Can you work these out from the drawing? Everything is in mm from the part's minimum corner. Give positions to 0.01 mm unless a question says otherwise; leave off trailing zeros. Loops run counter-clockwise (first coordinate to the right, second up) from the corner with the lowest first, then second, coordinate; pieces in that order, holes last. Notation, with made-up numbers: (-23.5, -19.5) -> (11.5, -19.5) arc R35 ccw to (11.5, 16.5) -> close; hole circle Ø3 at (5.5, 37). An arc over 180 degrees is marked (long way). Return JSON: item names as keys, results as strings. Group by question number.
Q1. Will these pins go through, and if not, where does the flat tip stop? pin 1 (3 mm diameter, centred on x = 9, y = 9, fed in from -Z); pin 2 (1.8 mm diameter, centred on x = 14.63, y = 5.75, fed in from +Z); pin 3 (3 mm diameter, centred on x = 12.5, z = 4, fed in from -Y) (3 decimals); pin 4 (3 mm diameter, centred on x = 6, z = 1.5, fed in from +Y).
Q2. Suppose I cut it at D-D, the plane y = 13.25. Please give me the cut outline in (x, z).
Q3. I need wall thicknesses on line 1 along Y through (x, z) = (9, 6.75); line 2 along X through (y, z) = (5.25, 6) (1 decimal); line 3 along X through (y, z) = (1.75, 4.5). Which ranges of each line are inside material? Lowest first, please. Write a range as [from, to].
Q4. Suppose I cut it at B-B, the plane y = 9. Please give me the cut outline in (x, z).
Q5. Thinking about a two-plate mould opening in Y: for the marked faces 1, 2 and 3, which applies, pulls with the +Y half, pulls with the -Y half, needs draft (parallel to the pull), parting line crosses it, or undercut?
Q6. Suppose I cut it at C-C, the plane z = 7. Please give me the cut outline in (x, y).
Q7. Suppose I cut it at A-A, the plane x = 9. Please give me the cut outline in (y, z), and give its area (3 significant figures).
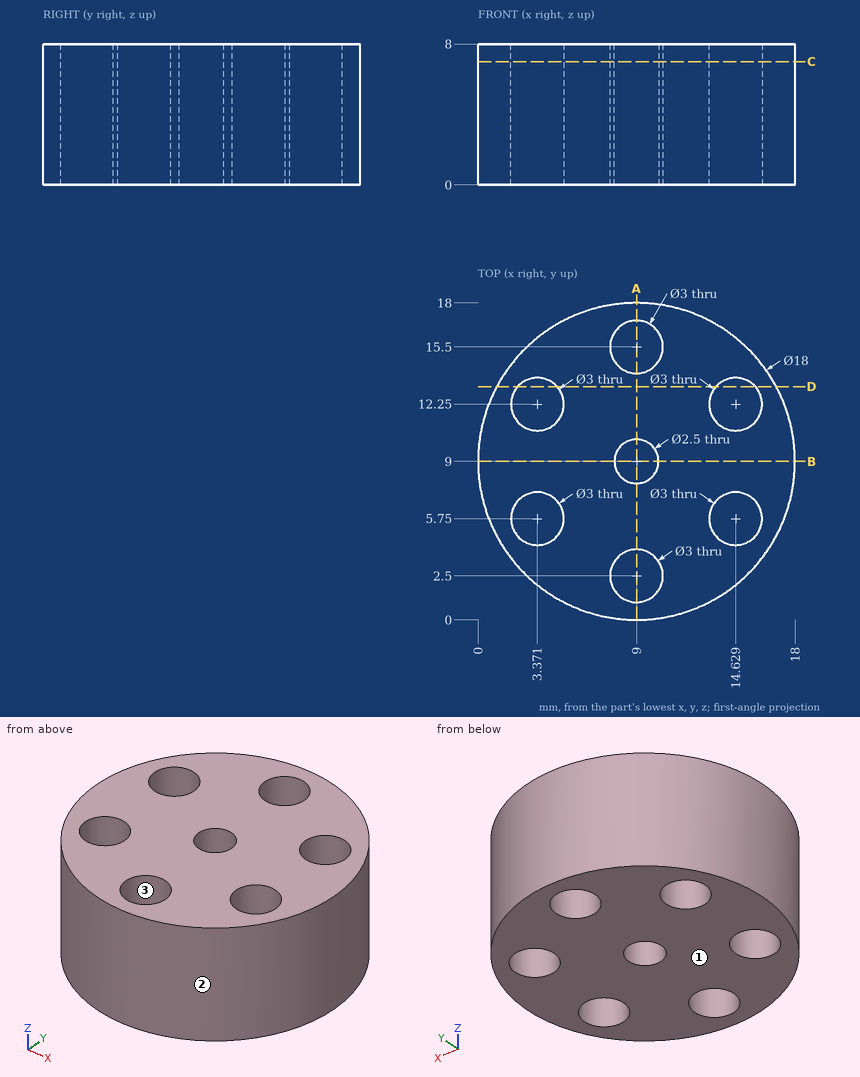
Ans:
{
 "1": {"pin 1": "stops at z = 0", "pin 2": "passes through", "pin 3": "stops at y = 0.225", "pin 4": "stops at y = 17.87"},
 "2": {"outline": "(1.07, 0) -> (2.25, 0) -> (2.25, 8) -> (1.07, 8) -> close; (4.49, 0) -> (13.51, 0) -> (13.51, 8) -> (4.49, 8) -> close; (15.75, 0) -> (16.93, 0) -> (16.93, 8) -> (15.75, 8) -> close"},
 "3": {"line 1": "y = [0, 1], [4, 7.75], [10.25, 14], [17, 18]", "line 2": "x = [0.8, 2], [4.8, 13.2], [16, 17.2]", "line 3": "x = [3.67, 7.7], [10.3, 14.33]"},
 "4": {"outline": "(0, 0) -> (7.75, 0) -> (7.75, 8) -> (0, 8) -> close; (10.25, 0) -> (18, 0) -> (18, 8) -> (10.25, 8) -> close"},
 "5": {"face 1": "needs draft", "face 2": "parting line crosses it", "face 3": "undercut"},
 "6": {"outline": "circle Ø18 at (9, 9); hole circle Ø3 at (3.37, 5.75); hole circle Ø3 at (3.37, 12.25); hole circle Ø3 at (9, 2.5); hole circle Ø3 at (9, 15.5); hole circle Ø2.5 at (9, 9); hole circle Ø3 at (14.63, 5.75); hole circle Ø3 at (14.63, 12.25)"},
 "7": {"outline": "(0, 0) -> (1, 0) -> (1, 8) -> (0, 8) -> close; (4, 0) -> (7.75, 0) -> (7.75, 8) -> (4, 8) -> close; (10.25, 0) -> (14, 0) -> (14, 8) -> (10.25, 8) -> close; (17, 0) -> (18, 0) -> (18, 8) -> (17, 8) -> close", "area": "76.0 mm^2"}
}
